Verification items for the finished model (mm, model axes). A direction names the side the tool comes from. Coordinates: 2 decimals unless noted, no trailing zeros. Order: outer loops, then holes, each group sorted by start corner. A loop starts at its lowest first (then second) coordinate and runs counter-clockwise, first axis right, second up. Notation, with made-up numbers: M 30.5,67 L 59.5,67 A6 ccw 59.5,72 Z; hole C -22,76.5 d10. An arc over 180 degrees is marked long. Return JSON: item names as keys, results as strings. Group by question number.
Q1. Thickness scan on probe 1 along X at (y, z) = (17.9, -25.45); probe 2 along Z at (x, y) = (2, 5.5); probe 3 along Y at (x, z) = (10.5, -12). Record the ranges inside material, lowest first.
Q2. Section check B-B, the plane z = 2.55. Enter the section's corners in (x, y), then the cut area to 3 significant figures.
Q3. Section check A-A, the plane z = -25.45. Enter the section's corners in (x, y).
Q4. Section check C-C, the plane y = 16.5. Enter the section's corners in (x, z).
Q5. Access from +Z, -Z, +X, -X, +Y, -Y to the whole of each face (thin tool, end or side, straight path). Record for faces 5 (the face through (4, 1, -24)), 6 (the face through (5.9, 18.6, 0.8)), 7 (the face through (11, 23.2, -22)).
Q6. Mould release check, pull along Z, two halves, no side actions. Record for faces 1 (the face through (6.05, 17.37, -23.95)), 2 (the face through (5.94, 25.22, -8.4)), 3 (the face through (6, 21, 0)), 4 (the face through (12, 11, -11)): pulls with the +Z half, pulls with the -Z half, needs draft (parallel to the pull), parting line crosses it, or undercut.
Q7. Go/stop test with flat-tipped pins: pin 1 Ø5.5 at (x, z) = (8, -25.5) entering from +Y; pin 2 Ø3.5 at (x, y) = (8, 21) entering from +Z; pin 3 Ø3.5 at (x, y) = (5, 2) entering from -Z; pin 4 Ø2.5 at (x, z) = (6, 2.55) entering from -Y. Record where each tip stops, or that it passes through.
Q8. Section check D-D, the plane x = 9.5. Enter the section's corners in (y, z).
from build123d import *

# Parameters (mm, degrees)
SKETCH_1_W          = 12
SKETCH_1_H          = 22.9
EXTRUDE_1_DEPTH     = 23.2
SKETCH_2_R          = 6
SKETCH_2_R_2        = 2
EXTRUDE_2_DEPTH     = 4.1
SKETCH_3_R          = 2.5
EXTRUDE_3_DEPTH     = 3
SKETCH_4_W          = 12
SKETCH_4_H          = 2.5
EXTRUDE_4_DEPTH     = 4.8
CUT_EXTRUDE_1_REACH = 33.849
SKETCH_6_W          = 2
SKETCH_6_H          = 3
EXTRUDE_5_DEPTH     = 3


with BuildPart() as part:
    # 草图1 → 凸台-拉伸1 (new body)
    with BuildSketch(Plane(origin=(0, 0, 0), x_dir=(1, 0, 0), z_dir=(0, 1, 0))):
        with Locations((6, 11.45)):
            Rectangle(SKETCH_1_W, SKETCH_1_H)
    extrude(amount=EXTRUDE_1_DEPTH)

    # 草图2 → 凸台-拉伸2 (add)
    with BuildSketch(Plane(origin=(0, 23.2, 0), x_dir=(1, 0, 0), z_dir=(0, 1, 0))):
        with Locations((6, 16.9)):
            Circle(SKETCH_2_R)
        with Locations((6, 10.4)):
            Circle(SKETCH_2_R_2)
    extrude(amount=EXTRUDE_2_DEPTH)

    # 草图3 → 凸台-拉伸3 (add)
    with BuildSketch(Plane(origin=(0, 27.3, 0), x_dir=(1, 0, 0), z_dir=(0, 1, 0))):
        with Locations(Location((6, 16.9, 0), (0, 0, 270))):
            Circle(SKETCH_3_R)
    extrude(amount=EXTRUDE_3_DEPTH)

    # 草图4 → 凸台-拉伸4 (add)
    with BuildSketch(Plane.XY):
        with Locations((6, 17.35)):
            Rectangle(SKETCH_4_W, SKETCH_4_H)
    extrude_4 = extrude(amount=EXTRUDE_4_DEPTH)

    # 草图5 → 切除-拉伸1 (cut, up to next)
    with BuildSketch(Plane(origin=(0, 18.6, 0), x_dir=(1, 0, 0), z_dir=(0, 1, 0)), mode=Mode.PRIVATE) as cut_extrude_1_sk1:
        with BuildLine():
            Line((5.25, -4.8), (6.75, -4.8))
            Line((6.75, -4.8), (6.75, -3.849038106))
            ThreePointArc((6.75, -3.849038106), (6, -1.05), (5.25, -3.849038106))
            Line((5.25, -3.849038106), (5.25, -4.8))
        make_face()
    cut_extrude_1_tool1 = extrude(cut_extrude_1_sk1.sketch, amount=-CUT_EXTRUDE_1_REACH, mode=Mode.PRIVATE) & part.part
    cut_extrude_1 = cut_extrude_1_tool1.solids().sort_by_distance((6, 18.6, 2.821372))[0]
    add(cut_extrude_1, mode=Mode.SUBTRACT)

    # 镜向1: 凸台-拉伸4, 切除-拉伸1 across plane
    add(extrude_4.mirror(Plane.XY.offset(-11.45)))
    add(cut_extrude_1.mirror(Plane.XY.offset(-11.45)), mode=Mode.SUBTRACT)

    # 草图6 → 凸台-拉伸5 (add)
    with BuildSketch(Plane(origin=(0, 0, -22.9), x_dir=(-1, 0, 0), z_dir=(0, 0, -1))):
        with Locations((-7, 1.5)):
            Rectangle(SKETCH_6_W, SKETCH_6_H)
        with Locations((-5, 1.5)):
            Rectangle(SKETCH_6_W, SKETCH_6_H)
    extrude(amount=EXTRUDE_5_DEPTH)


solid = part.part
Numbers:
{
 "1": {"probe 1": "x = 0 to 4.5, 7.5 to 12", "probe 2": "z = -22.9 to 0", "probe 3": "y = 0 to 23.2"},
 "2": {"outline": "M 0,16.1 L 4.5,16.1 L 4.5,18.6 L 0,18.6 Z; M 7.5,16.1 L 12,16.1 L 12,18.6 L 7.5,18.6 Z", "area": "22.5 mm2"},
 "3": {"outline": "M 0,16.1 L 4.5,16.1 L 4.5,18.6 L 0,18.6 Z; M 4,0 L 8,0 L 8,3 L 4,3 Z; M 7.5,16.1 L 12,16.1 L 12,18.6 L 7.5,18.6 Z"},
 "4": {"outline": "M 0,-27.7 L 5.25,-27.7 L 5.25,-26.75 A1.5 cw long 6.75,-26.75 L 6.75,-27.7 L 12,-27.7 L 12,4.8 L 6.75,4.8 L 6.75,3.85 A1.5 cw long 5.25,3.85 L 5.25,4.8 L 0,4.8 Z"},
 "5": {"face 5": "-Z, -X, -Y", "face 6": "+Z, +X, -X, +Y", "face 7": "-Z, +X, +Y"},
 "6": {"face 1": "undercut", "face 2": "undercut", "face 3": "pulls with the +Z half", "face 4": "needs draft"},
 "7": {"pin 1": "stops at y = 23.2", "pin 2": "stops at z = 0", "pin 3": "stops at z = -25.9", "pin 4": "passes through"},
 "8": {"outline": "M 0,-22.9 L 16.1,-22.9 L 16.1,-27.7 L 18.6,-27.7 L 18.6,-22.9 L 23.2,-22.9 L 23.2,-21.77 L 27.3,-21.77 L 27.3,-12.03 L 23.2,-12.03 L 23.2,0 L 18.6,0 L 18.6,4.8 L 16.1,4.8 L 16.1,0 L 0,0 Z"}
}
